Check sheet for the drawn part. Datum: minimum x, y, z corner. Units: mm. A direction names the side the tool comes from. Coordinates: 2 decimals unless noted, no trailing zeros. Loops run counter-clockwise (first coordinate to the right, second up) from the corner with the lowest first, then second, coordinate; pieces in that order, holes last.
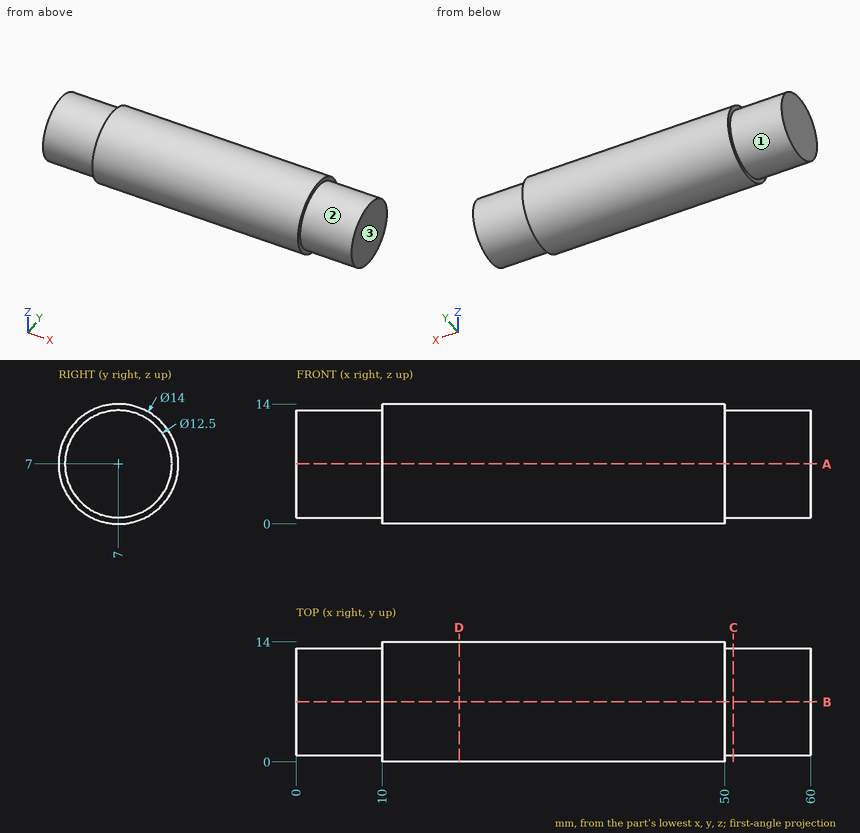
(1) Sectioned sample at A-A on z = 7. Record the cut outline in (x, y).
Findings:
outline: (0, 0.75) - (10, 0.75) - (10, 0) - (50, 0) - (50, 0.75) - (60, 0.75) - (60, 13.25) - (50, 13.25) - (50, 14) - (10, 14) - (10, 13.25) - (0, 13.25) - close
(2) Sectioned sample at D-D on x = 19. Record the cut outline in (y, z), and give its area (3 significant figures).
Findings:
outline: circle Ø14 at (7, 7)
area: 154 mm2
(3) Gauge pin test, flat ends, axial feed: pin 1 Ø8 at (x, z) = (36, 12) entering from -Y; pin 2 Ø5 at (x, z) = (51, 10) entering from -Y; pin 3 Ø1 at (x, z) = (34, 5.5) entering from +Y. Record the tip position at first contact, or that the pin passes through.
Findings:
pin 1: stops at y = 0.07
pin 2: stops at y = 0.04
pin 3: stops at y = 13.93
(4) Scan lines: L1, parallel to Y at x = 28.5, z = 8; L2, parallel to Z at x = 38, y = 9; L3, parallel to Y at x = 13.5, z = 5.5. Record each from-to range of solid material in increasing order.
Findings:
L1: y = 0.07 to 13.93
L2: z = 0.29 to 13.71
L3: y = 0.16 to 13.84
(5) Sectioned sample at C-C on x = 51. Record the cut outline in (y, z).
Findings:
outline: circle Ø12.5 at (7, 7)
(6) Access from +Z, -Z, +X, -X, +Y, -Y to the whole of each face (thin tool, end or side, straight path). Record for the marked faces 1, 2 and 3.
Findings:
face 1: -X
face 2: +X
face 3: +Z, -Z, +X, +Y, -Y
